Can you work these out from the model? Positions are in its coordinate system, mm. A direction names the side the tool comes from. Coordinates: 2 decimals unless noted, no trailing zeros. Order: outer loops, then holes, each group sorted by start corner. A loop starts at its lowest first (then second) coordinate and runs counter-clockwise, first axis right, second up. Notation, with made-up numbers: (-8, 2.5) -> (8, 2.5) arc R33 cw to (8, 36.5) -> close; hole circle Ø4 at (-8, -21). An arc over 180 degrees is marked (long way). Answer as CSV lines item,"result".
from build123d import *

# Parameters (mm, degrees)
SKETCH_1_W                     = 320
SKETCH_1_H                     = 58
EXTRUDE_1_DEPTH                = 20
SKETCH_2_W                     = 12
SKETCH_2_H                     = 1.5
CUT_EXTRUDE_1_DEPTH            = 326.828175577
HOLE_WIZARD_M6_1_D             = 5
HOLE_WIZARD_M6_1_DEPTH         = 15
HOLE_WIZARD_M6_1_TIP           = 1.502151548
HOLE_WIZARD_M6_1_2_D           = 7
HOLE_WIZARD_M6_1_2_CBORE_D     = 11
HOLE_WIZARD_M6_1_2_CBORE_DEPTH = 6
HOLE_WIZARD_M3_1_D             = 2.5
HOLE_WIZARD_M3_1_DEPTH         = 7.5
HOLE_WIZARD_M3_1_TIP           = 0.751075774
HOLE_WIZARD_M6_2_D             = 5
HOLE_WIZARD_M6_2_DEPTH         = 15
HOLE_WIZARD_M6_2_TIP           = 1.502151548
HOLE_WIZARD_M3_2_D             = 2.5
HOLE_WIZARD_M3_2_DEPTH         = 7.5
HOLE_WIZARD_M3_2_TIP           = 0.751075774


with BuildPart() as part:
    # 草图1 → 凸台-拉伸1 (new body)
    with BuildSketch(Plane.XY):
        with Locations((160, 29)):
            Rectangle(SKETCH_1_W, SKETCH_1_H)
    extrude(amount=EXTRUDE_1_DEPTH)

    # 草图2 → 切除-拉伸1 (cut, through all)
    with BuildSketch(Plane.ZY):
        with Locations((10, 57.25)):
            Rectangle(SKETCH_2_W, SKETCH_2_H)
    extrude(amount=-CUT_EXTRUDE_1_DEPTH, mode=Mode.SUBTRACT)

    # Hole Wizard M6 _1
    with Locations(Plane.XY.offset(20)):
        with Locations((160, 29), (150, 44)):
            Hole(HOLE_WIZARD_M6_1_D / 2, depth=HOLE_WIZARD_M6_1_DEPTH)
            with Locations((0, 0, -(HOLE_WIZARD_M6_1_DEPTH + HOLE_WIZARD_M6_1_TIP / 2))):  # 118° drill point
                Cone(0, HOLE_WIZARD_M6_1_D / 2, HOLE_WIZARD_M6_1_TIP, mode=Mode.SUBTRACT)

    # Hole Wizard M6 _1 2 (through all)
    with Locations(Plane(origin=(0, 56.5, 0), x_dir=(-1, 0, 0), z_dir=(0, 1, 0))):
        with Locations((-25, 10), (-295, 10), (-160, 10)):
            CounterBoreHole(HOLE_WIZARD_M6_1_2_D / 2, HOLE_WIZARD_M6_1_2_CBORE_D / 2, HOLE_WIZARD_M6_1_2_CBORE_DEPTH)

    # M3 螺纹孔1
    with Locations(Plane(origin=(0, 56.5, 0), x_dir=(-1, 0, 0), z_dir=(0, 1, 0))):
        with Locations((-265, 10), (-40, 10), (-190, 10), (-115, 10)):
            Hole(HOLE_WIZARD_M3_1_D / 2, depth=HOLE_WIZARD_M3_1_DEPTH)
            with Locations((0, 0, -(HOLE_WIZARD_M3_1_DEPTH + HOLE_WIZARD_M3_1_TIP / 2))):  # 118° drill point
                Cone(0, HOLE_WIZARD_M3_1_D / 2, HOLE_WIZARD_M3_1_TIP, mode=Mode.SUBTRACT)

    # M6 螺纹孔2
    with Locations(Plane(origin=(0, 0, 0), x_dir=(-1, 0, 0), z_dir=(0, 0, -1))):
        with Locations((-304, 46.621481833), (-276, 46.621481833)):
            Hole(HOLE_WIZARD_M6_2_D / 2, depth=HOLE_WIZARD_M6_2_DEPTH)
            with Locations((0, 0, -(HOLE_WIZARD_M6_2_DEPTH + HOLE_WIZARD_M6_2_TIP / 2))):  # 118° drill point
                Cone(0, HOLE_WIZARD_M6_2_D / 2, HOLE_WIZARD_M6_2_TIP, mode=Mode.SUBTRACT)

    # M3 螺纹孔2
    with Locations(Plane(origin=(0, 0, 0), x_dir=(-1, 0, 0), z_dir=(0, 0, -1))):
        with Locations((-10, 35.4), (-29.5, 35.4), (-244, 35.4), (-224.5, 35.4)):
            Hole(HOLE_WIZARD_M3_2_D / 2, depth=HOLE_WIZARD_M3_2_DEPTH)
            with Locations((0, 0, -(HOLE_WIZARD_M3_2_DEPTH + HOLE_WIZARD_M3_2_TIP / 2))):  # 118° drill point
                Cone(0, HOLE_WIZARD_M3_2_D / 2, HOLE_WIZARD_M3_2_TIP, mode=Mode.SUBTRACT)


solid = part.part
Q1. For P1, Ø6, axis at x = 276, y = 46.62, coming from the -Z side; P2, Ø3, axis at x = 40, z = 10, coming from the +Y side; P3, Ø5.5, axis at x = 158.5, z = 9.5, coming from the +Y side, each with a flat end and sliding along its axis, tell me the tip position at first contact or that it passes through.
Solution:
P1,"z = 0"
P2,"y = 56.5"
P3,"y = 50.5"
Q2. Which directions (+Z, -Z, +X, -X, +Y, -Y) give clear straight access to the entire face, cutting with the end or side of a thin tool? Please do faces 1 (the flat face through (157.8, 56.5, 4.6)), 2 (the cylindrical face through (306.309, 45.664, 7.605)), 3 (the flat face through (25, 50.5, 6)), 4 (the cylindrical face through (147.69, 43.04, 12.4)).
Solution:
face 1,"+X, -X, +Y"
face 2,"-Z"
face 3,"+Y"
face 4,"+Z"
Q3. If I drill on line 1 (X direction, y = 35.4, z = 4.75); line 2 (Y direction, x = 160, z = 6.35); line 3 (X direction, y = 20, z = 11), over which ranges is the centre line in solid material (lowest first)?
Solution:
line 1,"0 to 8.75, 11.25 to 28.25, 30.75 to 223.25, 225.75 to 242.75, 245.25 to 320"
line 2,"0 to 26.5, 31.5 to 50.5"
line 3,"0 to 21.65, 28.35 to 156.65, 163.35 to 291.65, 298.35 to 320"
Q4. Imagine slicing it at B-B (y = 5). List the corners of the cut face in (x, z) for me, and give its area (3 significant figures).
Solution:
outline,"(0, 0) -> (320, 0) -> (320, 20) -> (0, 20) -> close; hole circle Ø7 at (25, 10); hole circle Ø7 at (160, 10); hole circle Ø7 at (295, 10)"
area,"6,280 mm2"
Q5. Imagine slicing it at C-C (x = 119). List the corners of the cut face in (y, z) for me, and give its area (3 significant figures).
Solution:
outline,"(0, 0) -> (58, 0) -> (58, 4) -> (56.5, 4) -> (56.5, 16) -> (58, 16) -> (58, 20) -> (0, 20) -> close"
area,"1,140 mm2"
Q6. We'd pull the mould along Z, two halves only. Please class faces 5 (the flat face through (160, 50.5, 6)), 6 (the cylindrical face through (278.309, 45.664, 7.605)), 7 (the conical face through (304.32, 46.915, 16.241)), 8 (the flat face through (291, 50.5, 10)): pulls with the +Z half, pulls with the -Z half, needs draft (parallel to the pull), parting line crosses it, or undercut.
Solution:
face 5,"undercut"
face 6,"needs draft"
face 7,"pulls with the -Z half"
face 8,"undercut"
Q7. Imagine slicing it at A-A (x = 25). List the corners of the cut face in (y, z) for me, and give its area (4 significant figures).
Solution:
outline,"(0, 0) -> (58, 0) -> (58, 4) -> (56.5, 4) -> (56.5, 4.5) -> (50.5, 4.5) -> (50.5, 6.5) -> (0, 6.5) -> close; (0, 13.5) -> (50.5, 13.5) -> (50.5, 15.5) -> (56.5, 15.5) -> (56.5, 16) -> (58, 16) -> (58, 20) -> (0, 20) -> close"
area,"722.5 mm2"
